from build123d import *

# Parameters (mm, degrees)
SKETCH1_W           = 160
SKETCH1_H           = 50
BOSS_EXTRUDE1_DEPTH = 10
SKETCH2_W           = 10
SKETCH2_H           = 50
BOSS_EXTRUDE2_DEPTH = 50
SKETCH3_W           = 9.9
SKETCH3_H           = 29.9
BOSS_EXTRUDE3_DEPTH = 10


with BuildPart() as part:
    # Sketch1 → Boss-Extrude1 (new body)
    with BuildSketch(Plane(origin=(0, 0, 0), x_dir=(1, 0, 0), z_dir=(0, 1, 0))):
        Rectangle(SKETCH1_W, SKETCH1_H)
    extrude(amount=BOSS_EXTRUDE1_DEPTH)

    # Sketch2 → Boss-Extrude2 (add)
    with BuildSketch(Plane(origin=(0, 10, 0), x_dir=(1, 0, 0), z_dir=(0, 1, 0))):
        with Locations((-75, 0)):
            Rectangle(SKETCH2_W, SKETCH2_H)
        with Locations((75, 0)):
            Rectangle(SKETCH2_W, SKETCH2_H)
    extrude(amount=BOSS_EXTRUDE2_DEPTH)

    # Sketch3 → Boss-Extrude3 (add)
    with BuildSketch(Plane(origin=(0, 60, 0), x_dir=(1, 0, 0), z_dir=(0, 1, 0))):
        with Locations((-75, 0)):
            Rectangle(SKETCH3_W, SKETCH3_H)
        with Locations((75, 0)):
            Rectangle(SKETCH3_W, SKETCH3_H)
    extrude(amount=BOSS_EXTRUDE3_DEPTH)


solid = part.part
Model file for the job. Use its own axes, mm. A direction names the side the tool comes from. Round coordinates to 2 decimals unless told otherwise and drop trailing zeros. Order: outer loops, then holes, each group sorted by start corner. A loop starts at its lowest first (then second) coordinate and runs counter-clockwise, first axis right, second up.
(1) Band-saw the part on D-D (y = 15). List the corners of the cut face in (x, z), then the cut area to 3 significant figures.
(2) Pin check, flat tips, straight feed: pin 1 (5 mm diameter, centred on y = 66, z = -1.5, fed in from +X); pin 2 (2 mm diameter, centred on x = 54.5, z = 14.5, fed in from +Y); pin 3 (3 mm diameter, centred on x = -76.5, y = 64.5, fed in from -Z). Stop position of each tip, or through.
(3) Band-saw the part on C-C (x = -54). List the corners of the cut face in (y, z).
(4) Band-saw the part on A-A (y = 65.5). List the corners of the cut face in (x, z), then the cut area to 3 significant figures.
(5) Band-saw the part on B-B (z = 20). List the corners of the cut face in (x, y).
(6) Pull direction X, two halves, no side cores. Call faces 1 (the face through (75, 65, -14.95)), 2 (the face through (70.05, 65, 0)), 3 (the face through (79.95, 65, 0)): released by +X, released by -X, zero draft, split by the parting line, or undercut.
(7) Drill centre lines: line 1 (X direction, y = 29, z = -4); line 2 (Y direction, x = 50, z = -7). Where is each one in solid material? Low to high.
(8) 3-axis set-ups, long thin cutter, end or side, ignore diameter. For faces 4 (the face through (75, 65, 14.95)), 5 (the face through (70, 35, 0)), 6 (the face through (-75, 65, -14.95)): which of +Z, -Z, +X, -X, +Y, -Y reach the whole face in a straight line?
Verdict:
1. outline: (-80, -25) - (-70, -25) - (-70, 25) - (-80, 25) - close; (70, -25) - (80, -25) - (80, 25) - (70, 25) - close
1. area: 1,000 mm2
2. pin 1: stops at x = 79.95
2. pin 2: stops at y = 10
2. pin 3: stops at z = -14.95
3. outline: (0, -25) - (10, -25) - (10, 25) - (0, 25) - close
4. outline: (-79.95, -14.95) - (-70.05, -14.95) - (-70.05, 14.95) - (-79.95, 14.95) - close; (70.05, -14.95) - (79.95, -14.95) - (79.95, 14.95) - (70.05, 14.95) - close
4. area: 592 mm2
5. outline: (-80, 0) - (80, 0) - (80, 60) - (70, 60) - (70, 10) - (-70, 10) - (-70, 60) - (-80, 60) - close
6. face 1: zero draft
6. face 2: undercut
6. face 3: released by +X
7. line 1: x = -80 to -70, 70 to 80
7. line 2: y = 0 to 10
8. face 4: +Z, +X, -X, +Y
8. face 5: +Z, -Z, +Y
8. face 6: -Z, +X, -X, +Y
